from build123d import *

# Parameters (mm, degrees)
SKETCH1_W           = 203.2
SKETCH1_H           = 101.6
BOSS_EXTRUDE1_DEPTH = 3.175
SKETCH2_W           = 3.175
SKETCH2_H           = 12.7
SKETCH2_W_2         = 25.4
SKETCH2_H_2         = 6.35
BOSS_EXTRUDE2_DEPTH = 3.175
SKETCH3_W           = 25.4
SKETCH3_H           = 6.35
CUT_EXTRUDE1_DEPTH  = 120.947785411


with BuildPart() as part:
    # Sketch1 → Boss-Extrude1 (new body)
    with BuildSketch(Plane.XY):
        Rectangle(SKETCH1_W, SKETCH1_H)
    extrude(amount=BOSS_EXTRUDE1_DEPTH)

    # Sketch2 → Boss-Extrude2 (add)
    with BuildSketch(Plane.XY.offset(3.175)):
        with Locations((-103.1875, 19.05)):
            Rectangle(SKETCH2_W, SKETCH2_H)
        with Locations((-103.1875, 44.45)):
            Rectangle(SKETCH2_W, SKETCH2_H)
        with Locations((-103.1875, -6.35)):
            Rectangle(SKETCH2_W, SKETCH2_H)
        with Locations((-103.1875, -31.75)):
            Rectangle(SKETCH2_W, SKETCH2_H)
        with Locations((-92.075, -53.975)):
            Rectangle(SKETCH2_W_2, SKETCH2_H_2)
        with Locations((-30.48, -53.975)):
            Rectangle(SKETCH2_W_2, SKETCH2_H_2)
        with Locations((31.115, -53.975)):
            Rectangle(SKETCH2_W_2, SKETCH2_H_2)
        with Locations((92.71, -53.975)):
            Rectangle(SKETCH2_W_2, SKETCH2_H_2)
        with Locations((103.1875, -31.75)):
            Rectangle(SKETCH2_W, SKETCH2_H)
        with Locations((103.1875, -6.35)):
            Rectangle(SKETCH2_W, SKETCH2_H)
        with Locations((103.1875, 19.05)):
            Rectangle(SKETCH2_W, SKETCH2_H)
        with Locations((103.1875, 44.45)):
            Rectangle(SKETCH2_W, SKETCH2_H)
    extrude(amount=-BOSS_EXTRUDE2_DEPTH)

    # Sketch3 → Cut-Extrude1 (cut, through all)
    with BuildSketch(Plane.XY.offset(3.175)):
        with Locations((-92.075, -53.975)):
            Rectangle(SKETCH3_W, SKETCH3_H)
        with Locations((92.71, -53.975)):
            Rectangle(SKETCH3_W, SKETCH3_H)
    extrude(amount=-CUT_EXTRUDE1_DEPTH, mode=Mode.SUBTRACT)


solid = part.part
Model file for the job. Use its own axes, mm. Coordinates: 2 decimals unless noted, no trailing zeros. Order: outer loops, then holes, each group sorted by start corner. A loop starts at its lowest first (then second) coordinate and runs counter-clockwise, first axis right, second up. Notation, with made-up numbers: (86, 56) -> (92, 56) arc R13 cw to (92, 70) -> close; hole circle Ø8 at (29.25, 20). An arc over 180 degrees is marked (long way). Return JSON: item names as keys, results as strings. Group by question number.
Item 1: Flat gauge pins, fed straight in: P1, Ø1.6, axis at y = -43, z = 1, coming from the -X side; P2, Ø1.6, axis at x = -104, z = 2, coming from the -Y side; P3, Ø1, axis at x = 73, z = 1, coming from the -Y side. Where does each tip first touch, or does it go through?
Item 2: Saw through at B-B on y = -45. Write the cut outline in (x, z) (3 decimals), then the cut area to 3 significant figures.
Item 3: Wall check: line 1 along Y through (x, z) = (70, 1); line 2 along X through (y, z) = (-47, 1.35). Give the ranges that are in metal, low to high. Write a range as [from, to].
Item 4: Saw through at A-A on x = 70.5. Write the cut outline in (y, z) (3 decimals), then the cut area to 3 significant figures.
Values found:
{
 "1": {"P1": "stops at x = -101.6", "P2": "stops at y = -38.1", "P3": "stops at y = -50.8"},
 "2": {"outline": "(-101.6, 0) -> (101.6, 0) -> (101.6, 3.175) -> (-101.6, 3.175) -> close", "area": "645 mm2"},
 "3": {"line 1": "y = [-50.8, 50.8]", "line 2": "x = [-101.6, 101.6]"},
 "4": {"outline": "(-50.8, 0) -> (50.8, 0) -> (50.8, 3.175) -> (-50.8, 3.175) -> close", "area": "323 mm2"}
}
